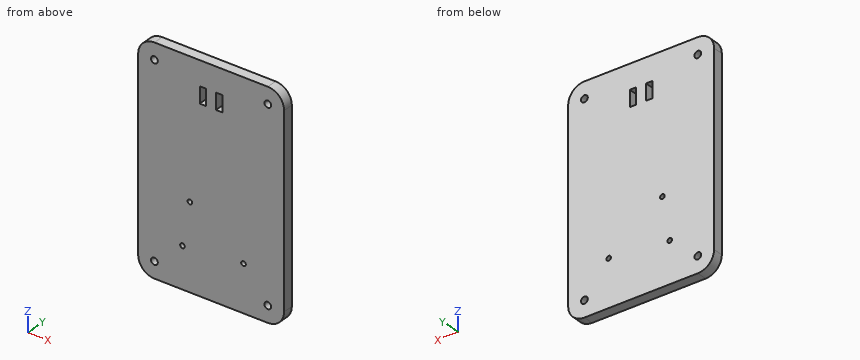
```python
from build123d import *

# Parameters (mm, degrees)
SKETCH1_R           = 2.0828
SKETCH1_R_2         = 1.4224
SKETCH1_W           = 4
SKETCH1_H           = 10
BOSS_EXTRUDE1_DEPTH = 6.35


with BuildPart() as part:
    # Sketch1 → Boss-Extrude1 (new body)
    with BuildSketch(Plane(origin=(0, 0, 0), x_dir=(1, 0, 0), z_dir=(0, 1, 0))):
        with BuildLine():
            Line((-34.925, -67.912), (34.925, -67.912))
            ThreePointArc((34.925, -67.912), (41.996067812, -64.983067812), (44.925, -57.912))
            Line((44.925, -57.912), (44.925, 57.912))
            ThreePointArc((44.925, 57.912), (41.996067812, 64.983067812), (34.925, 67.912))
            Line((34.925, 67.912), (-34.925, 67.912))
            ThreePointArc((-34.925, 67.912), (-41.996067812, 64.983067812), (-44.925, 57.912))
            Line((-44.925, 57.912), (-44.925, -57.912))
            ThreePointArc((-44.925, -57.912), (-41.996067812, -64.983067812), (-34.925, -67.912))
        make_face()
        with Locations(Location((-34.925, 57.912, 0), (0, 0, 270))):
            Circle(SKETCH1_R, mode=Mode.SUBTRACT)
        with Locations(Location((34.925, 57.912, 0), (0, 0, 270))):
            Circle(SKETCH1_R, mode=Mode.SUBTRACT)
        with Locations(Location((34.925, -57.912, 0), (0, 0, 270))):
            Circle(SKETCH1_R, mode=Mode.SUBTRACT)
        with Locations(Location((-34.925, -57.912, 0), (0, 0, 270))):
            Circle(SKETCH1_R, mode=Mode.SUBTRACT)
        with Locations(Location((19.939, 39.276, 0), (0, 0, 270))):
            Circle(SKETCH1_R_2, mode=Mode.SUBTRACT)
        with Locations(Location((-13.081, 15.8572, 0), (0, 0, 270))):
            Circle(SKETCH1_R_2, mode=Mode.SUBTRACT)
        with Locations(Location((-17.653, 42.705, 0), (0, 0, 270))):
            Circle(SKETCH1_R_2, mode=Mode.SUBTRACT)
        with Locations((-5, -47.912)):
            Rectangle(SKETCH1_W, SKETCH1_H, mode=Mode.SUBTRACT)
        with Locations((5, -47.912)):
            Rectangle(SKETCH1_W, SKETCH1_H, mode=Mode.SUBTRACT)
    extrude(amount=BOSS_EXTRUDE1_DEPTH)


solid = part.part
```
The listing builds one solid part. Answer for the finished solid, in the listing's coordinates (mm). Round coordinates to 2 decimals unless told otherwise and drop trailing zeros. Loops run counter-clockwise (first coordinate to the right, second up) from the corner with the lowest first, then second, coordinate; pieces in that order, holes last. Notation, with made-up numbers: (86, 8.5) - (99, 8.5) arc R31 cw to (99, 34.5) - close; hole circle Ø9 at (38, 88). An arc over 180 degrees is marked (long way). Use one line per item in the form item = value. Start each with the question number.
1. Consider line 1 (Z direction, x = -4, y = 2.5); line 2 (Z direction, x = 38.5, y = 1.75); line 3 (Z direction, x = 41, y = 5.75). Determine where each line is inside the solid, lowest interval first. Write a range as [from, to].
2. The part is cut by section C-C on x = 39.5. Determine the outline of the cut face in (y, z).
3. Given pin 1 Ø3.5 at (x, z) = (34.925, -57.912) entering from +Y, flat-ended and moving along its own axis, determine where the tip first touches the part or whether it passes through.
4. The part is cut by section B-B on y = 3.75. Give the number of separate pieces and of enclosed holes in the cut face, then the cut area to 3 significant figures.
5. The part is cut by section A-A on z = 46. Determine the outline of the cut face in (x, y) (3 decimals).
Geometry check:
q1.line_1 = [-67.91, 42.91], [52.91, 67.91]
q1.line_2 = [-67.25, 67.25]
q1.line_3 = [-65.86, 65.86]
q2.outline = (0, -66.8) - (6.35, -66.8) - (6.35, 66.8) - (0, 66.8) - close
q3.pin_1 = through
q4.separate_pieces = 1
q4.enclosed_holes = 9
q4.area = 12,000 mm^2
q5.outline = (-44.925, 0) - (-7, 0) - (-7, 6.35) - (-44.925, 6.35) - close; (-3, 0) - (3, 0) - (3, 6.35) - (-3, 6.35) - close; (7, 0) - (44.925, 0) - (44.925, 6.35) - (7, 6.35) - close
